The model under review builds one solid part; all positions refer to its coordinate system, in mm. A direction names the side the tool comes from. Give positions to 0.01 mm unless a question says otherwise; leave off trailing zeros. Order: outer loops, then holes, each group sorted by start corner. A loop starts at its lowest first (then second) coordinate and runs counter-clockwise, first axis right, second up. Notation, with made-up numbers: M -5,14 L 41,14 A22 ccw 41,48 Z; hole C 55.5,47.25 d6. An arc over 180 degrees is marked long. One line per question, with ' | ' between items. Start each with the question number.
1. We need section B-B on x = 0. Write out the cut boundary in (y, z), then the cut area to 3 significant figures.
2. For faces 5 (the face through (17.746, -0.182, 5.505)), 6 (the face through (-22.8, 0.2, 6)), list the 3-axis set-ups (+Z, -Z, +X, -X, +Y, -Y) from which the entire face can be reached by the end or side of a thin tool; tool diameter is ignored.
3. We need section D-D on z = 14. Write out the cut boundary in (x, y), then the cut area to 3 significant figures.
4. Insertion check: P1, Ø6.5, axis at x = 0, y = 0, coming from the +Z side; P2, Ø2, axis at y = 5, z = 5, coming from the +X side; P3, Ø4, axis at y = -3.5, z = 11.5, coming from the +X side. Each pin has a flat end and moves straight along its axis. Give the tip position at first contact, or say it passes through.
5. Wall thickness on L1, parallel to Y at x = 0, z = 8; L2, parallel to X at y = 1.5, z = 8.75; L3, parallel to X at y = -2, z = 10: over which ranges is each line inside the solid? List them lowest first.
6. We need section A-A on y = 0. Count the separate pieces of the cut face and the enclosed holes in it, then the cut area to 3 significant figures.
7. We need section C-C on x = 21. Write out the cut boundary in (y, z).
8. The part is to be moulded in two halves that separate along Y. For faces 1 (the face through (-1, 13, 8)), 2 (the face through (25.6, -0.18, 13.72)), 3 (the face through (-23.323, 2.103, 2.958)), 4 (the face through (-19.81, -4.21, 11.07)), say which applies: +Y half, -Y half, draft (parallel to the pull), parting line (faces both ways), or undercut.
```python
from build123d import *

# Parameters (mm, degrees)
SKETCH002_R  = 11
PAD002_DEPTH = 10
SKETCH001_R  = 4.1
PAD001_DEPTH = 26
SKETCH_R     = 7
SKETCH_R_2   = 3.95
PAD_DEPTH    = 16
FILLET_R     = 7.99


with BuildPart() as pad002:
    # Sketch002 → Pad002 (new body)
    with BuildSketch(Plane.XY.offset(16)):
        with Locations((-29.971518, 0)):
            Circle(SKETCH002_R)
    extrude(amount=-PAD002_DEPTH)


with BuildPart() as cutblock:
    # Sketch001 → Pad001 (new body)
    with BuildSketch(Plane.XZ.offset(13)):
        with Locations((21, 8)):
            Circle(SKETCH001_R)
    extrude(amount=-PAD001_DEPTH)

    # Fusion: union Pad002
    add(pad002.part)


with BuildPart() as fillet_body:
    # Sketch → Pad (new body)
    with BuildSketch(Plane.XY):
        with BuildLine():
            ThreePointArc((-30, 13), (-43, 0), (-30, -13))
            Line((-30, -13), (28, -13))
            Line((28, 13), (28, -13))
            Line((-30, 13), (28, 13))
        make_face()
        with Locations((-30, 0)):
            Circle(SKETCH_R, mode=Mode.SUBTRACT)
        Circle(SKETCH_R_2, mode=Mode.SUBTRACT)
    extrude(amount=PAD_DEPTH)

    # Cut: cut CutBlock
    add(cutblock.part, mode=Mode.SUBTRACT)

    # Fillet
    fillet_edges = [fillet_body.edges().sort_by_distance(p)[0] for p in [
        (28, 0, 16),
        (28, 0, 0),
    ]]
    fillet(fillet_edges, radius=FILLET_R)


solid = fillet_body.part
```
Entries:
1) outline: M -13,0 L -3.95,0 L -3.95,16 L -13,16 Z; M 3.95,0 L 13,0 L 13,16 L 3.95,16 Z | area: 290 mm^2
2) face 5: +Y, -Y | face 6: +Z
3) outline: M -30,-13 L 25.3,-13 L 25.3,13 L -30,13 A13 ccw Z; hole C -29.97,0 d22; hole C 0,0 d7.9 | area: 1,270 mm^2
4) P1: passes through | P2: stops at x = 27.75 | P3: stops at x = 27.86
5) L1: y = -13 to -3.95, 3.95 to 13 | L2: x = -42.91 to -40.87, -19.07 to -3.65, 3.65 to 16.97, 25.03 to 27.97 | L3: x = -42.85 to -40.79, -19.15 to -3.41, 3.41 to 17.42, 24.58 to 27.75
6) separate pieces: 3 | enclosed holes: 1 | area: 625 mm^2
7) outline: M -13,0.06 L 13,0.06 L 13,3.9 L -13,3.9 Z; M -13,12.1 L 13,12.1 L 13,15.94 L -13,15.94 Z
8) face 1: +Y half | face 2: draft | face 3: undercut | face 4: undercut
